Verification items for the finished model (mm, model axes). Face numbers are marked on the shaded views. Coordinates: 2 decimals unless noted, no trailing zeros. Order: outer loops, then holes, each group sorted by start corner. A loop starts at its lowest first (then second) coordinate and runs counter-clockwise, first axis right, second up. Notation, with made-up numbers: M 54.25,71.25 L 101.25,71.25 A23 ccw 101.25,103.25 Z; hole C -14,-17.75 d2. An arc over 180 degrees is marked long. Return JSON: item names as keys, results as strings. Group by question number.
Q1. Section check B-B, the plane y = 4. Enter the section's corners in (x, z).
Q2. Mould release check, pull along X, two halves, no side actions. Record for the marked faces 1, 2, 3 and 4: pulls with the +X half, pulls with the -X half, needs draft (parallel to the pull), parting line crosses it, or undercut.
Q3. Section check A-A, the plane y = 0. Enter the section's corners in (x, z), then the cut area to 4 significant figures.
Q4. Thickness scan on probe 1 along X at (y, z) = (-0.25, 1.15); probe 2 along X at (y, z) = (-1.75, 1.1); probe 3 along Y at (x, z) = (51.5, 1.3). Record the ranges inside material, lowest first.
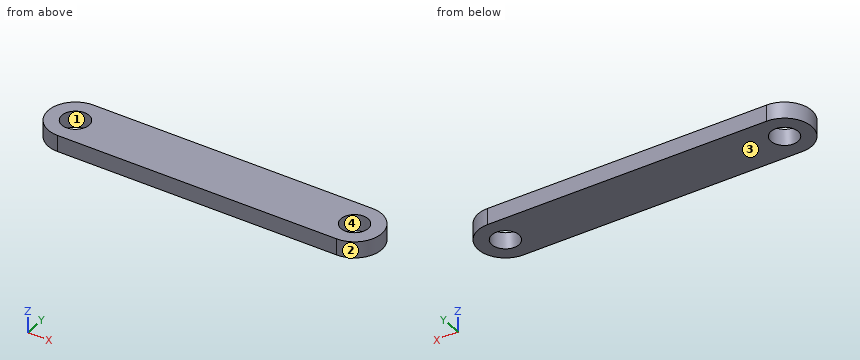
Autodesk Inventor part; units mm, degrees
ref_plane "YZ Plane" through (0, 0, 0) normal (1, 0, 0) x (0, 1, 0)
ref_plane "XZ Plane" through (0, 0, 0) normal (0, 1, 0) x (-1, 0, 0)
ref_plane "XY Plane" through (0, 0, 0) normal (0, 0, 1) x (1, 0, 0)
sketch "草圖1" plane through (0, 0, 0) normal (0, 0, 1) x (1, 0, 0)
  line L0 (0, 0) -> (51.5, 0) construction
  line L1 (0, -5) -> (51.5, -5)
  line L2 (51.5, 5) -> (0, 5)
  arc A0 (0, 5) -> (0, -5) centre (0, 0) ccw
  arc A1 (51.5, -5) -> (51.5, 5) centre (51.5, 0) ccw
  point P0 (25.75, 0)
  dimension "d0" = 51.5
  dimension "d1" = 5
extrude "擠出1" add sketch "草圖1" along normal blind 3
hole "孔1" at (51.5, 0, 3) direction (0, 0, -1) diameter 5 depth 8 tip angle 118
hole "孔2" at (0, 0, 3) direction (0, 0, -1) diameter 5 depth 8 tip angle 118
properties part number "02連桿25"
Numbers:
{
 "1": {"outline": "M -3,0 L 54.5,0 L 54.5,3 L -3,3 Z"},
 "2": {"face 1": "undercut", "face 2": "pulls with the +X half", "face 3": "needs draft", "face 4": "undercut"},
 "3": {"outline": "M -5,0 L -2.5,0 L -2.5,3 L -5,3 Z; M 2.5,0 L 49,0 L 49,3 L 2.5,3 Z; M 54,0 L 56.5,0 L 56.5,3 L 54,3 Z", "area": "154.5 mm2"},
 "4": {"probe 1": "x = -4.99 to -2.49, 2.49 to 49.01, 53.99 to 56.49", "probe 2": "x = -4.68 to -1.79, 1.79 to 49.71, 53.29 to 56.18", "probe 3": "y = -5 to -2.5, 2.5 to 5"}
}
